from build123d import *

# Parameters (mm, degrees)
SKETCH_1_R           = 2.5
SKETCH_1_R_2         = 1
EXTRUDE_1_DEPTH      = 2
SKETCH_2_R           = 3.5
SKETCH_2_R_2         = 2.5
EXTRUDE_2_DEPTH      = 2
EXTRUDE_3_DEPTH      = 0.1
EXTRUDE_3_DEPTH_BACK = 0.1
SKETCH_3_R           = 2.5
SKETCH_3_R_2         = 1.5


with BuildPart() as part:
    # 草圖1 → 填料-伸長1 (new body)
    with BuildSketch(Plane(origin=(0, 0, 0), x_dir=(1, 0, 0), z_dir=(0, 1, 0))):
        with BuildLine():
            Line((-9.444444444, 1.949992086), (-0.888888889, 3.899984172))
            ThreePointArc((-0.888888889, 3.899984172), (0, 4), (0.888888889, 3.899984172))
            Line((0.888888889, 3.899984172), (9.444444444, 1.949992086))
            ThreePointArc((9.444444444, 1.949992086), (11, 0), (9.444444444, -1.949992086))
            Line((9.444444444, -1.949992086), (0.888888889, -3.899984172))
            ThreePointArc((0.888888889, -3.899984172), (0, -4), (-0.888888889, -3.899984172))
            Line((-0.888888889, -3.899984172), (-9.444444444, -1.949992086))
            ThreePointArc((-9.444444444, -1.949992086), (-11, 0), (-9.444444444, 1.949992086))
        make_face()
        with Locations(Location((0, 0, 0), (0, 0, 270))):
            Circle(SKETCH_1_R, mode=Mode.SUBTRACT)
        with Locations(Location((-9, 0, 0), (0, 0, 270))):
            Circle(SKETCH_1_R_2, mode=Mode.SUBTRACT)
        with Locations(Location((9, 0, 0), (0, 0, 270))):
            Circle(SKETCH_1_R_2, mode=Mode.SUBTRACT)
    extrude(amount=EXTRUDE_1_DEPTH)

    # 草圖2 → 填料-伸長2 (add)
    with BuildSketch(Plane(origin=(0, 2, 0), x_dir=(1, 0, 0), z_dir=(0, 1, 0))):
        with Locations(Location((0, 0, 0), (0, 0, 270))):
            Circle(SKETCH_2_R)
        with Locations(Location((0, 0, 0), (0, 0, 270))):
            Circle(SKETCH_2_R_2, mode=Mode.SUBTRACT)
    extrude(amount=EXTRUDE_2_DEPTH)

    # 草圖3 → 填料-伸長3 (add, two sides: drawn at the far end of the back side and taken through both)
    with BuildSketch(Plane(origin=(0, 2, 0), x_dir=(1, 0, 0), z_dir=(0, 1, 0)).offset(-EXTRUDE_3_DEPTH_BACK)):
        with Locations(Location((0, 0, 0), (0, 0, 270))):
            Circle(SKETCH_3_R)
        with Locations(Location((0, 0, 0), (0, 0, 270))):
            Circle(SKETCH_3_R_2, mode=Mode.SUBTRACT)
    extrude(amount=EXTRUDE_3_DEPTH + EXTRUDE_3_DEPTH_BACK)


solid = part.part
Verification items for the finished model (mm, model axes). A direction names the side the tool comes from. Round coordinates to 2 decimals unless told otherwise and drop trailing zeros. Loops run counter-clockwise (first coordinate to the right, second up) from the corner with the lowest first, then second, coordinate; pieces in that order, holes last. Notation, with made-up numbers: M 88.5,21 L 132.5,21 A13 ccw 132.5,35 Z; hole C 11.5,30 d11. An arc over 180 degrees is marked long. Write each question's results on one line, items separated by ' | '.
1) Access from +Z, -Z, +X, -X, +Y, -Y to the whole of each face (thin tool, end or side, straight path). Record for faces 1 (the cylindrical face through (-3.417, 2.986, -0.759)), 2 (the flat face through (5.107, 0.986, -2.939)), 3 (the cylindrical face through (-2.44, 0.94, -0.54)).
Checks:
face 1: +Y | face 2: -Z, +X, +Y, -Y | face 3: -Y
2) Scan lines: L1, parallel to X at y = 2.8, z = 0; L2, parallel to Y at x = 7.75, z = -2.25; L3, parallel to X at y = 1.5, z = -0.5. Record each from-to range of solid material in increasing order. Write a range as from..to.
Checks:
L1: x = -3.5..-2.5, 2.5..3.5 | L2: y = 0..2 | L3: x = -10.94..-9.87, -8.13..-2.45, 2.45..8.13, 9.87..10.94
3) Section check B-B on z = 0. Record the boundary of the cut face in (x, y).
Checks:
outline: M -11,0 L -10,0 L -10,2 L -11,2 Z; M -8,0 L -2.5,0 L -2.5,1.9 L -1.5,1.9 L -1.5,2.1 L -2.5,2.1 L -2.5,4 L -3.5,4 L -3.5,2 L -8,2 Z; M 1.5,1.9 L 2.5,1.9 L 2.5,0 L 8,0 L 8,2 L 3.5,2 L 3.5,4 L 2.5,4 L 2.5,2.1 L 1.5,2.1 Z; M 10,0 L 11,0 L 11,2 L 10,2 Z
4) Section check A-A on x = 0. Record the boundary of the cut face in (y, z).
Checks:
outline: M 0,-4 L 2,-4 L 2,-3.5 L 4,-3.5 L 4,-2.5 L 2.1,-2.5 L 2.1,-1.5 L 1.9,-1.5 L 1.9,-2.5 L 0,-2.5 Z; M 0,2.5 L 1.9,2.5 L 1.9,1.5 L 2.1,1.5 L 2.1,2.5 L 4,2.5 L 4,3.5 L 2,3.5 L 2,4 L 0,4 Z
5) Mould release check, pull along X, two halves, no side actions. Record for faces 4 (the flat face through (0, 0, 3)), 5 (the cylindrical face through (0, 1, -4)), 6 (the flat face through (-2, 1.9, 0)): released by +X, released by -X, zero draft, split by the parting line, or undercut.
Checks:
face 4: zero draft | face 5: split by the parting line | face 6: undercut
6) Section check C-C on y = 1. Record the boundary of the cut face in (x, z), then the cut area to 3 significant figures.
Checks:
outline: M -9.44,-1.95 L -0.89,-3.9 A4 ccw 0.89,-3.9 L 9.44,-1.95 A2 ccw 9.44,1.95 L 0.89,3.9 A4 ccw -0.89,3.9 L -9.44,1.95 A2 ccw Z; hole C -9,0 d2; hole C 0,0 d5; hole C 9,0 d2 | area: 97.3 mm2
7) Gauge pin test, flat ends, axial feed: P1, Ø1, axis at x = -3.5, z = 2.5, coming from the +Y side; P2, Ø1.5, axis at y = 3.5, z = -2, coming from the -X side. Record the tip position at first contact, or that the pin passes through.
Checks:
P1: stops at y = 2 | P2: stops at x = -3.27
8) Section check D-D on z = -1.25. Record the boundary of the cut face in (x, y).
Checks:
outline: M -10.56,0 L -2.17,0 L -2.17,1.9 L -0.83,1.9 L -0.83,2.1 L -2.17,2.1 L -2.17,4 L -3.27,4 L -3.27,2 L -10.56,2 Z; M 0.83,1.9 L 2.17,1.9 L 2.17,0 L 10.56,0 L 10.56,2 L 3.27,2 L 3.27,4 L 2.17,4 L 2.17,2.1 L 0.83,2.1 Z
